For this review, use the dimensioned drawing (mm, ordinates from the lowest corner) and the shaded views. A direction names the side the tool comes from. Round coordinates to 2 decimals unless told otherwise and drop trailing zeros. Write each loop counter-clockwise with the first axis right and the second up, starting at its lowest first coordinate (ties: lowest second). Pieces come first, ordered by that corner, then holes. Notation, with made-up numbers: M 69,12.25 L 127,12.25 A30 ccw 127,50.25 Z; hole C 30,31.25 d3. An arc over 180 degrees is marked long. One line per question, with ' | ' between items. Start each with the question number.
Item 1: Machinability: for the marked faces 4 and 5, which of the approach directions +Z, -Z, +X, -X, +Y, -Y give a long, thin tool a straight path to every point of the face, cutting with its end or side? Answer none if there is none.
Item 2: Add section B-B, the plane x = 13.5. State the section outline as (y, z) points, and give its area (3 significant figures).
Item 3: Add section D-D, the plane z = 28.25. State the section outline as (x, y) points, and give its area (3 significant figures).
Item 4: Draft analysis for pull direction Z (two halves, no side actions). For the marked faces 1, 2 and 3, state which applies: released by +Z, released by -Z, zero draft, split by the parting line, or undercut.
Item 5: Insertion check: pin 1 Ø3 at (x, z) = (4, 17.5) entering from -Y; pin 2 Ø1.8 at (x, z) = (24, 16.5) entering from -Y; pin 3 Ø12 at (x, z) = (13.5, 10) entering from +Y. Each pin has a flat end and moves straight along its axis. Give the tip position at first contact, or say it passes through.
Item 6: Add section C-C, the plane y = 0.8. State the section outline as (x, z) points.
Item 7: For L1, parallel to X at y = 5.1, z = 17.5; L2, parallel to X at y = 1.3, z = 17.5; L3, parallel to Z at x = 17.75, y = 4.5 (1 decimal), list the stretches that pass through material, from the lowest coordinate up.
Item 8: Add section A-A, the plane z = 6.75. State the section outline as (x, y) points, and give its area (3 significant figures).
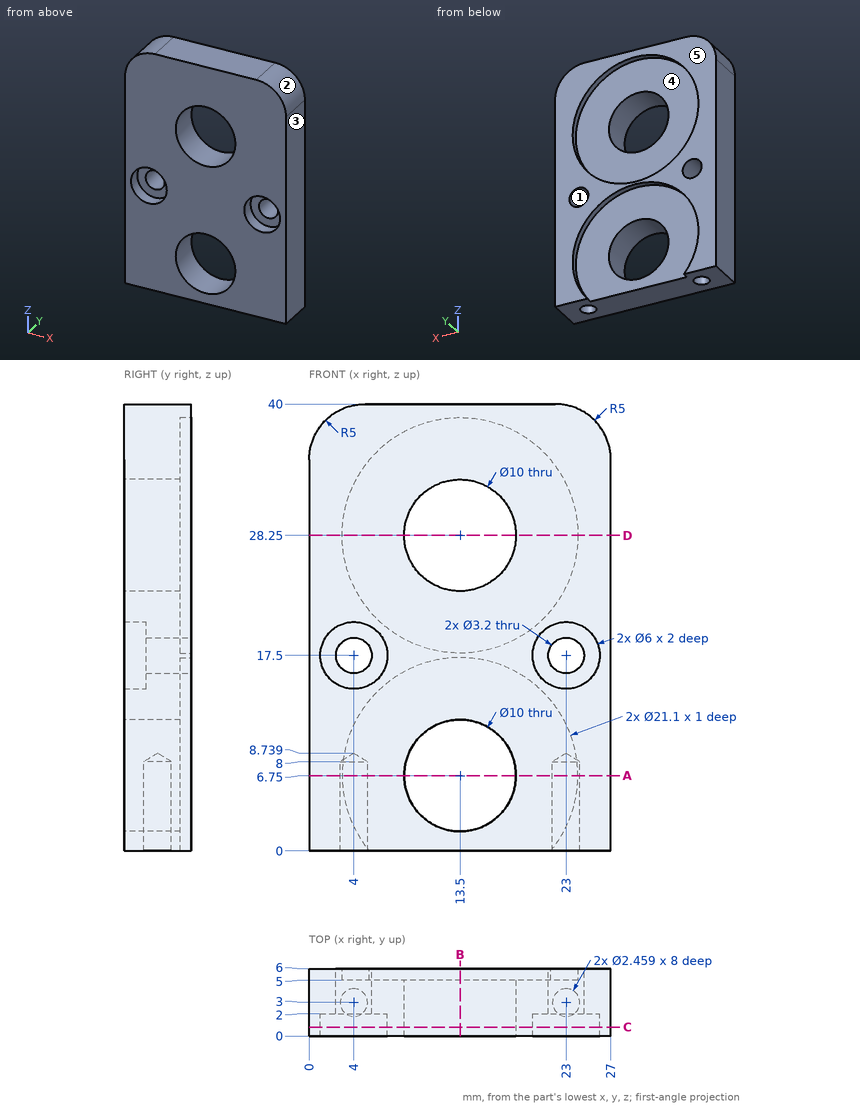
Computed values:
1) face 4: +Y | face 5: +Z, -Z, +X, -X, +Y
2) outline: M 0,0 L 5,0 L 5,1.75 L 0,1.75 Z; M 0,11.75 L 5,11.75 L 5,17.3 L 6,17.3 L 6,17.7 L 5,17.7 L 5,23.25 L 0,23.25 Z; M 0,33.25 L 5,33.25 L 5,38.8 L 6,38.8 L 6,40 L 0,40 Z | area: 102 mm^2
3) outline: M 0,0 L 8.5,0 L 8.5,5 L 2.95,5 L 2.95,6 L 0,6 Z; M 18.5,0 L 27,0 L 27,6 L 24.05,6 L 24.05,5 L 18.5,5 Z | area: 90.9 mm^2
4) face 1: undercut | face 2: released by +Z | face 3: zero draft
5) pin 1: passes through | pin 2: stops at y = 2 | pin 3: stops at y = 5
6) outline: M 0,0 L 27,0 L 27,35 A5 ccw 22,40 L 5,40 A5 ccw 0,35 Z; hole C 4,17.5 d6; hole C 13.5,6.75 d10; hole C 13.5,28.25 d10; hole C 23,17.5 d6
7) L1: x = 0 to 2.4, 5.6 to 21.4, 24.6 to 27 | L2: x = 0 to 1, 7 to 20, 26 to 27 | L3: z = 0 to 4.1, 9.4 to 25.6, 30.9 to 40
8) outline: M 0,0 L 8.5,0 L 8.5,5 L 2.95,5 L 2.95,6 L 0,6 Z; M 18.5,0 L 27,0 L 27,6 L 24.05,6 L 24.05,5 L 18.5,5 Z; hole C 4,3 d2.46; hole C 23,3 d2.46 | area: 81.4 mm^2
